Build history of the part. All positions in model axes, mm. A direction names the side the tool comes from. Round coordinates to 2 decimals unless told otherwise and drop trailing zeros. Answer as a JSON object with one key per item and string values.
from build123d import *

# Parameters (mm, degrees)
SKETCH_1_R      = 2.5
EXTRUDE_1_DEPTH = 300
EXTRUDE_START   = -300
SKETCH_2_W      = 8
SKETCH_2_H      = 8
SKETCH_2_R      = 2.5
EXTRUDE_2_DEPTH = 300
FILLET_1_R      = 1


with BuildPart() as part:
    # 草图1 → 凸台-拉伸1 (new body)
    with BuildSketch(Plane.XY):
        with BuildLine():
            Line((173.5, -150), (168.5, -150))
            Line((168.5, -150), (168.5, -150.5))
            Line((168.5, -150.5), (168, -150.5))
            Line((168, -150.5), (168, -151.70000008))
            Line((168, -151.70000008), (170.299390173, -151.70000008))
            ThreePointArc((170.299390173, -151.70000008), (170.94610582, -152.132121658), (170.794364905, -152.894974776))
            Line((170.794364905, -152.894974776), (167.175465502, -156.513874235))
            ThreePointArc((167.175465502, -156.513874235), (166.907085014, -156.653013019), (166.607569506, -156.61204781))
            ThreePointArc((166.607569506, -156.61204781), (165.969708818, -156.377547161), (165.299999837, -156.262019281))
            Line((165.299999837, -156.262019281), (165, -156.549999889))
            Line((165, -156.549999889), (164.700000163, -156.262019281))
            ThreePointArc((164.700000163, -156.262019281), (164.030290989, -156.377547213), (163.392430134, -156.61204798))
            ThreePointArc((163.392430134, -156.61204798), (163.092914607, -156.653013217), (162.824534093, -156.513874431))
            Line((162.824534093, -156.513874431), (159.205634442, -152.89497478))
            ThreePointArc((159.205634442, -152.89497478), (159.053893522, -152.13212166), (159.70060917, -151.70000008))
            Line((159.70060917, -151.70000008), (162, -151.70000008))
            Line((162, -151.70000008), (162, -150.5))
            Line((162, -150.5), (161.500000104, -150.5))
            Line((161.500000104, -150.5), (161.500000104, -150))
            Line((161.500000104, -150), (156.500000104, -150))
            ThreePointArc((156.500000104, -150), (155.439339932, -150.439339828), (155.000000104, -151.5))
            Line((155.000000104, -151.5), (155.000000104, -156.5))
            Line((155.000000104, -156.5), (155.500000104, -156.5))
            Line((155.500000104, -156.5), (155.500000104, -157))
            Line((155.500000104, -157), (156.699999897, -157))
            Line((156.699999897, -157), (156.699999897, -154.700608431))
            ThreePointArc((156.699999897, -154.700608431), (157.132121491, -154.053892778), (157.894974619, -154.205633725))
            Line((157.894974619, -154.205633725), (161.513874525, -157.824533943))
            ThreePointArc((161.513874525, -157.824533943), (161.653013299, -158.092914462), (161.61204805, -158.392429988))
            ThreePointArc((161.61204805, -158.392429988), (161.377547255, -159.030290833), (161.262019293, -159.700000002))
            Line((161.262019293, -159.700000002), (161.550000032, -160))
            Line((161.550000032, -160), (161.262019293, -160.299999998))
            ThreePointArc((161.262019293, -160.299999998), (161.37754719, -160.969708925), (161.612047835, -161.607569559))
            ThreePointArc((161.612047835, -161.607569559), (161.653013049, -161.907085066), (161.513874269, -162.175465556))
            Line((161.513874269, -162.175465556), (157.894974601, -165.79436528))
            ThreePointArc((157.894974601, -165.79436528), (157.13212148, -165.946106205), (156.699999897, -165.299390557))
            Line((156.699999897, -165.299390557), (156.699999897, -163))
            Line((156.699999897, -163), (155.500000104, -163))
            Line((155.500000104, -163), (155.500000104, -163.5))
            Line((155.500000104, -163.5), (155.000000104, -163.5))
            Line((155.000000104, -163.5), (155.000000104, -168.5))
            ThreePointArc((155.000000104, -168.5), (155.439339932, -169.560660172), (156.500000104, -170))
            Line((156.500000104, -170), (161.500000104, -170))
            Line((161.500000104, -170), (161.500000104, -169.5))
            Line((161.500000104, -169.5), (162, -169.5))
            Line((162, -169.5), (162, -168.29999992))
            Line((162, -168.29999992), (159.700610052, -168.29999992))
            ThreePointArc((159.700610052, -168.29999992), (159.053894408, -167.867878348), (159.205635312, -167.105025232))
            Line((159.205635312, -167.105025232), (162.824534559, -163.486125803))
            ThreePointArc((162.824534559, -163.486125803), (163.092915044, -163.346987014), (163.392430553, -163.387952218))
            ThreePointArc((163.392430553, -163.387952218), (164.030291195, -163.622452842), (164.700000125, -163.737980716))
            Line((164.700000125, -163.737980716), (165, -163.450000078))
            Line((165, -163.450000078), (165.299999781, -163.737980724))
            ThreePointArc((165.299999781, -163.737980724), (165.969708906, -163.622452815), (166.60756972, -163.387952089))
            ThreePointArc((166.60756972, -163.387952089), (166.907085249, -163.346986865), (167.175465757, -163.486125663))
            Line((167.175465757, -163.486125663), (170.794365024, -167.105025241))
            ThreePointArc((170.794365024, -167.105025241), (170.946105917, -167.867878353), (170.299390275, -168.29999992))
            Line((170.299390275, -168.29999992), (168, -168.29999992))
            Line((168, -168.29999992), (168, -169.5))
            Line((168, -169.5), (168.5, -169.5))
            Line((168.5, -169.5), (168.5, -170))
            Line((168.5, -170), (173.5, -170))
            ThreePointArc((173.5, -170), (174.560660172, -169.560660172), (175, -168.5))
            Line((175, -168.5), (175, -163.5))
            Line((175, -163.5), (174.499999896, -163.5))
            Line((174.499999896, -163.5), (174.499999896, -163))
            Line((174.499999896, -163), (173.300000103, -163))
            Line((173.300000103, -163), (173.300000103, -165.299391013))
            ThreePointArc((173.300000103, -165.299391013), (172.867878523, -165.946106661), (172.105025403, -165.794365741))
            Line((172.105025403, -165.794365741), (168.486125569, -162.175465907))
            ThreePointArc((168.486125569, -162.175465907), (168.346986783, -161.907085393), (168.38795202, -161.607569866))
            ThreePointArc((168.38795202, -161.607569866), (168.622452774, -160.969709062), (168.737980711, -160.299999942))
            Line((168.737980711, -160.299999942), (168.450000002, -160))
            Line((168.450000002, -160), (168.73798071, -159.70000004))
            ThreePointArc((168.73798071, -159.70000004), (168.622452807, -159.030291062), (168.387952137, -158.392430382))
            ThreePointArc((168.387952137, -158.392430382), (168.346986918, -158.092914876), (168.486125693, -157.824534383))
            Line((168.486125693, -157.824534383), (172.10502539, -154.205634503))
            ThreePointArc((172.10502539, -154.205634503), (172.867878514, -154.053893567), (173.300000103, -154.700609218))
            Line((173.300000103, -154.700609218), (173.300000103, -157))
            Line((173.300000103, -157), (174.499999896, -157))
            Line((174.499999896, -157), (174.499999896, -156.5))
            Line((174.499999896, -156.5), (175, -156.5))
            Line((175, -156.5), (175, -151.5))
            ThreePointArc((175, -151.5), (174.560660172, -150.439339828), (173.5, -150))
        make_face()
        with Locations((165, -160)):
            Circle(SKETCH_1_R, mode=Mode.SUBTRACT)
    extrude(amount=EXTRUDE_1_DEPTH)

    # 草图2 → 凸台-拉伸2 (add)
    with BuildSketch(Plane.XY.offset(300).offset(EXTRUDE_START)):
        with Locations((165, -160)):
            Rectangle(SKETCH_2_W, SKETCH_2_H)
        with Locations((165, -160)):
            Circle(SKETCH_2_R, mode=Mode.SUBTRACT)
    extrude(amount=EXTRUDE_2_DEPTH)

    # 圆角1
    fillet_1_edges = [part.edges().sort_by_distance(p)[0] for p in [
        (169, -157.31066005, 150),
        (167.68934005, -164, 150),
        (161, -162.689339833, 150),
        (162.310659662, -156, 150),
        (167.689339729, -156, 150),
        (161, -157.310659374, 150),
        (162.310660387, -164, 150),
        (169, -162.689340338, 150),
    ]]
    fillet(fillet_1_edges, radius=FILLET_1_R)


solid = part.part
1) Flat gauge pins, fed straight in: pin 1 Ø3.5 at (x, z) = (165, 219) entering from -Y; pin 2 Ø0.6 at (y, z) = (-170, 82) entering from -X; pin 3 Ø1.4 at (y, z) = (-160.5, 99.5) entering from -X; pin 4 Ø3 at (x, y) = (165, -160) entering from -Z. Where does each tip first touch, or does it go through?
Checked values:
{"pin 1": "stops at y = -164", "pin 2": "stops at x = 155.6", "pin 3": "stops at x = 161", "pin 4": "passes through"}
2) Pull direction Y, two halves, no side cores. Call faces 1 (the face through (165, -164, 148)), 2 (the face through (161, -160, 148)), 3 (the face through (175, -154, 148)): pulls with the +Y half, pulls with the -Y half, needs draft (parallel to the pull), parting line crosses it, or undercut.
Checked values:
{"face 1": "pulls with the -Y half", "face 2": "undercut", "face 3": "needs draft"}
3) Which spindle directions (+Z, -Z, +X, -X, +Y, -Y) get a long thin tool onto all of the face, cutting with end or side? Do faces 4 (the face through (159, -170, 148)), 5 (the face through (169, -160, 148)), 6 (the face through (165, -156, 148)). Say none if no direction does.
Checked values:
{"face 4": "+Z, -Z, +X, -X, -Y", "face 5": "+Z, -Z, +X", "face 6": "+Z, -Z, +Y"}
4) Probe L1, parallel to X at y = -159.75, z = 168; L2, parallel to X at y = -155, z = 238; L3, parallel to X at y = -155.25, z = 193. List the from-to ranges inside material, lowest first. Write a range as from..to.
Checked values:
{"L1": "x = 161..162.51, 167.49..169", "L2": "x = 155..156.7, 158.69..161.31, 168.69..171.31, 173.3..175", "L3": "x = 155..156.7, 158.94..161.56, 168.44..171.06, 173.3..175"}
